Verification items for the finished model (mm, model axes). Face numbers are marked on the shaded views. Coordinates: 2 decimals unless noted, no trailing zeros. Write each loop counter-clockwise with the first axis right and the second up, starting at its lowest first coordinate (ties: lowest second). Pieces come first, ordered by that corner, then holes. Notation, with made-up numbers: (8.5, 10.25) -> (36.5, 10.25) arc R22 cw to (36.5, 23.25) -> close; hole circle Ø3 at (73, -8). An arc over 180 degrees is marked (long way). Write each question's results on one line, items separated by ' | '. Start each with the question number.
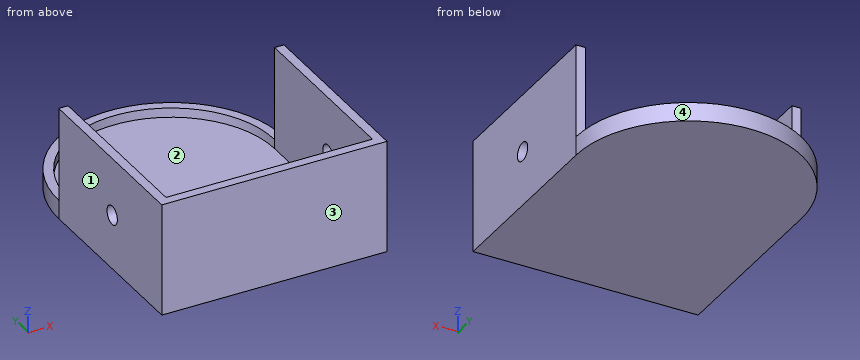
from build123d import *

# Parameters (mm, degrees)
F1_DEPTH = 3.175
F2_DEPTH = 6.35
F3_DEPTH = 38.1
F0_W     = 3.175
F0_H     = 60.325
F4_DEPTH = 38.1
F5_DEPTH = 38.1
F6_R     = 3.175
F7_DEPTH = 76.2


with BuildPart() as f1:
    # F0 (on Top) → F1 (new body)
    with BuildSketch(Plane.XY):
        with BuildLine():
            Line((34.925, -60.325), (34.925, 0))
            ThreePointArc((34.925, 0), (0, 34.925), (-34.925, 0))
            Line((-34.925, 0), (-34.925, -60.325))
            Line((-34.925, -60.325), (34.925, -60.325))
        make_face()
    extrude(amount=F1_DEPTH)

    # F0 (on Top) → F2 (join)
    with BuildSketch(Plane.XY):
        with BuildLine():
            Line((34.925, 0), (38.1, 0))
            ThreePointArc((38.1, 0), (0, 38.1), (-38.1, 0))
            Line((-38.1, 0), (-34.925, 0))
            ThreePointArc((-34.925, 0), (0, 34.925), (34.925, 0))
        make_face()
    extrude(amount=F2_DEPTH)

    # F0 (on Top) → F3 (join)
    with BuildSketch(Plane.XY):
        Polygon((38.1, -63.5), (38.1, -60.325), (34.925, -60.325), (-34.925, -60.325), (-38.1, -60.325), (-38.1, -63.5), align=None)
    extrude(amount=F3_DEPTH)

    # F0 (on Top) → F4 (join)
    with BuildSketch(Plane.XY):
        with Locations((-36.5125, -30.1625)):
            Rectangle(F0_W, F0_H)
    extrude(amount=F4_DEPTH)

    # F0 (on Top) → F5 (join)
    with BuildSketch(Plane.XY):
        with Locations((36.5125, -30.1625)):
            Rectangle(F0_W, F0_H)
    extrude(amount=F5_DEPTH)

    # F6 (on face) → F7 (cut)
    with BuildSketch(Plane.YZ.offset(38.1)):
        with Locations((-32.936446, 18.498553)):
            Circle(F6_R)
    extrude(amount=-F7_DEPTH, mode=Mode.SUBTRACT)


solid = f1.part
1. Mould release check, pull along X, two halves, no side actions. Record for the marked faces 1, 2, 3 and 4: +X half, -X half, draft (parallel to the pull), parting line (faces both ways), or undercut.
2. Sectioned sample at B-B on z = 10. Record the cut outline in (x, y) (3 decimals), plus the area to 3 significant figures.
3. Material ranges on probe 1 along X at (y, z) = (-39, 27.5) (3 decimals); probe 2 along Z at (x, y) = (-14.5, -14) (3 decimals); probe 3 along Y at (x, z) = (25, 11.5) (3 decimals), recorded low to high. Write a range as from..to.
4. Sectioned sample at A-A on y = -21.5. Record the cut outline in (x, z) (3 decimals), plus the area to 3 significant figures.
5. Depth check by flat-ended pin: pin 1 Ø5 at (x, y) = (-1.5, -50) entering from +Z (3 decimals); pin 2 Ø3.5 at (x, z) = (-37, 21) entering from +Y. Enter the tip coordinate at first touch or a pass-through.
Computed values:
1) face 1: -X half | face 2: undercut | face 3: draft | face 4: parting line
2) outline: (-38.1, -63.5) -> (38.1, -63.5) -> (38.1, 0) -> (34.925, 0) -> (34.925, -60.325) -> (-34.925, -60.325) -> (-34.925, 0) -> (-38.1, 0) -> close | area: 625 mm^2
3) probe 1: x = -38.1..-34.925, 34.925..38.1 | probe 2: z = 0..3.175 | probe 3: y = -63.5..-60.325
4) outline: (-38.1, 0) -> (38.1, 0) -> (38.1, 38.1) -> (34.925, 38.1) -> (34.925, 3.175) -> (-34.925, 3.175) -> (-34.925, 38.1) -> (-38.1, 38.1) -> close | area: 464 mm^2
5) pin 1: stops at z = 3.175 | pin 2: stops at y = 0
